from build123d import *

# Parameters (mm, degrees)
SKETCH1_W           = 67
SKETCH1_H           = 30
BOSS_EXTRUDE1_DEPTH = 25
SKETCH2_W           = 57
SKETCH2_H           = 22
CUT_EXTRUDE1_DEPTH  = 17
SKETCH3_R           = 10
SKETCH3_R_2         = 8
SKETCH3_R_3         = 2
CUT_EXTRUDE2_DEPTH  = 8
BOSS_EXTRUDE2_START = -67
SKETCH4_W           = 5
SKETCH4_H           = 15
BOSS_EXTRUDE2_DEPTH = 10
SKETCH4_2_W         = 5
SKETCH4_2_H         = 15
BOSS_EXTRUDE3_DEPTH = 10
SKETCH5_R           = 1.7
CUT_EXTRUDE3_DEPTH  = 10
CUT_EXTRUDE4_DEPTH  = 8
SKETCH8_W           = 67
SKETCH8_H           = 25
BOSS_EXTRUDE4_DEPTH = 50
SKETCH9_W           = 57
SKETCH9_H           = 22
CUT_EXTRUDE6_DEPTH  = 17
SKETCH11_R          = 10
SKETCH11_R_2        = 8
SKETCH11_R_3        = 2
CUT_EXTRUDE7_DEPTH  = 81.039052968
CUT_EXTRUDE8_DEPTH  = 81.039052968
FILLET1_R           = 3


with BuildPart() as part:
    # Sketch1 → Boss-Extrude1 (new body)
    with BuildSketch(Plane(origin=(0, 0, 0), x_dir=(1, 0, 0), z_dir=(0, 1, 0))):
        Rectangle(SKETCH1_W, SKETCH1_H)
    extrude(amount=BOSS_EXTRUDE1_DEPTH)

    # Sketch2 → Cut-Extrude1 (cut)
    with BuildSketch(Plane(origin=(0, 25, 0), x_dir=(1, 0, 0), z_dir=(0, 1, 0))):
        Rectangle(SKETCH2_W, SKETCH2_H)
    extrude(amount=-CUT_EXTRUDE1_DEPTH, mode=Mode.SUBTRACT)

    # Sketch3 → Cut-Extrude2 (cut)
    with BuildSketch(Plane(origin=(0, 8, 0), x_dir=(1, 0, 0), z_dir=(0, 1, 0))):
        with Locations((10, 0)):
            Circle(SKETCH3_R)
        with Locations((-3, 0)):
            Circle(SKETCH3_R_2)
        with Locations(Location((-24.5, 5, 0), (0, 0, 270))):
            Circle(SKETCH3_R_3)
        with Locations(Location((-24.5, -5, 0), (0, 0, 270))):
            Circle(SKETCH3_R_3)
        with Locations(Location((24.5, 5, 0), (0, 0, 270))):
            Circle(SKETCH3_R_3)
        with Locations(Location((24.5, -5, 0), (0, 0, 270))):
            Circle(SKETCH3_R_3)
    extrude(amount=-CUT_EXTRUDE2_DEPTH, mode=Mode.SUBTRACT)

    # Sketch4 → Boss-Extrude2 (add)
    with BuildSketch(Plane(origin=(33.5, 0, 0), x_dir=(0, 0, -1), z_dir=(1, 0, 0)).offset(BOSS_EXTRUDE2_START)):
        with Locations((-12.5, 12.5)):
            Rectangle(SKETCH4_W, SKETCH4_H)
    extrude(amount=-BOSS_EXTRUDE2_DEPTH)

    # Sketch4<2> → Boss-Extrude3 (add)
    with BuildSketch(Plane(origin=(33.5, 0, 0), x_dir=(0, 0, -1), z_dir=(1, 0, 0))):
        with Locations((-12.5, 12.5)):
            Rectangle(SKETCH4_2_W, SKETCH4_2_H)
    extrude(amount=BOSS_EXTRUDE3_DEPTH)

    # Sketch5 → Cut-Extrude3 (cut)
    with BuildSketch(Plane(origin=(0, 0, 10), x_dir=(-1, 0, 0), z_dir=(0, 0, -1))):
        with Locations(Location((38, 12.5, 0), (0, 0, 90))):
            Circle(SKETCH5_R)
        with Locations(Location((-38, 12.5, 0), (0, 0, 90))):
            Circle(SKETCH5_R)
    extrude(amount=-CUT_EXTRUDE3_DEPTH, mode=Mode.SUBTRACT)

    # Sketch6 → Cut-Extrude4 (cut)
    with BuildSketch(Plane(origin=(0, 8, 0), x_dir=(1, 0, 0), z_dir=(0, 1, 0))):
        Polygon((-21, 11.00455557), (-21.003329437, -10.997477388), (10, -11.002168937), (10, 10.997831063), align=None)
    extrude(amount=-CUT_EXTRUDE4_DEPTH, mode=Mode.SUBTRACT)

    # Sketch8 → Boss-Extrude4 (add)
    with BuildSketch(Plane(origin=(0, 0, -15), x_dir=(-1, 0, 0), z_dir=(0, 0, -1))):
        with Locations((0, 12.5)):
            Rectangle(SKETCH8_W, SKETCH8_H)
    extrude(amount=BOSS_EXTRUDE4_DEPTH)

    # Sketch9 → Cut-Extrude6 (cut)
    with BuildSketch(Plane(origin=(0, 25, 0), x_dir=(1, 0, 0), z_dir=(0, 1, 0))):
        with Locations((0, 30)):
            Rectangle(SKETCH9_W, SKETCH9_H)
    extrude(amount=-CUT_EXTRUDE6_DEPTH, mode=Mode.SUBTRACT)

    # Sketch11 → Cut-Extrude7 (cut, through all)
    with BuildSketch(Plane(origin=(0, 8, 0), x_dir=(1, 0, 0), z_dir=(0, 1, 0))):
        with Locations((9.177125898, 30.121191818)):
            Circle(SKETCH11_R)
        with Locations((-3.822874102, 30.121191818)):
            Circle(SKETCH11_R_2)
        with Locations(Location((-25.322874102, 35.121191818, 0), (0, 0, 270))):
            Circle(SKETCH11_R_3)
        with Locations(Location((-25.322874102, 25.121191818, 0), (0, 0, 270))):
            Circle(SKETCH11_R_3)
        with Locations(Location((23.677125898, 35.121191818, 0), (0, 0, 270))):
            Circle(SKETCH11_R_3)
        with Locations(Location((23.677125898, 25.121191818, 0), (0, 0, 270))):
            Circle(SKETCH11_R_3)
    extrude(amount=-CUT_EXTRUDE7_DEPTH, mode=Mode.SUBTRACT)

    # Sketch13 → Cut-Extrude8 (cut, through all)
    with BuildSketch(Plane(origin=(0, 8, 0), x_dir=(1, 0, 0), z_dir=(0, 1, 0))):
        Polygon((-20.928820676, 40.842619331), (-20.932150113, 18.840586374), (10.071179324, 18.835894824), (10.071179324, 40.835894824), align=None)
    extrude(amount=-CUT_EXTRUDE8_DEPTH, mode=Mode.SUBTRACT)

    # Fillet1
    fillet1_edges = [part.edges().sort_by_distance(p)[0] for p in [
        (0, 25, -41),
        (0, 25, -19),
        (0, 25, 11),
        (-43.5, 12.5, 10),
        (-33.5, 20, 12.5),
        (-33.5, 5, 12.5),
        (0, 25, -11),
        (33.5, 20, 12.5),
        (33.5, 5, 12.5),
        (43.5, 12.5, 10),
        (33.5, 12.5, -65),
        (-33.5, 12.5, -65),
    ]]
    fillet(fillet1_edges, radius=FILLET1_R)


solid = part.part
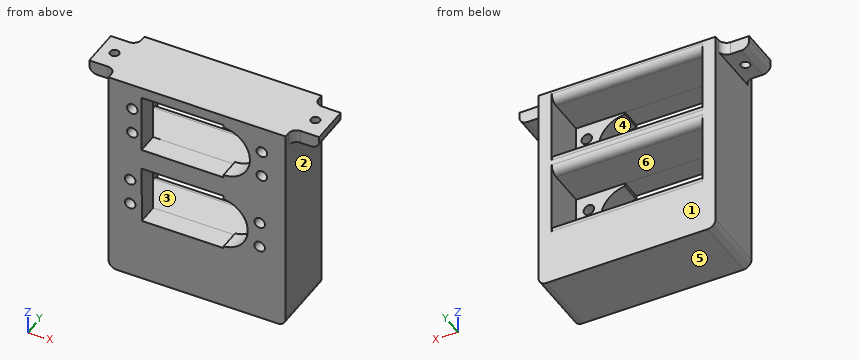
Build history of the part. All positions in model axes, mm. Face numbers are marked on the shaded views. A direction names the side the tool comes from. Round coordinates to 2 decimals unless told otherwise and drop trailing zeros. Loops run counter-clockwise (first coordinate to the right, second up) from the corner with the lowest first, then second, coordinate; pieces in that order, holes last. Notation, with made-up numbers: (50, 36) -> (99, 36) arc R24 cw to (99, 74) -> close; hole circle Ø9 at (-15, 19). An arc over 180 degrees is marked (long way). One line per item, written item: value. Start each with the question number.
Q1. Probe line 1 along Z through (x, y) = (-16, 11.25); line 2 along X through (y, z) = (12.5, 13.55); line 3 along Z through (x, y) = (2.5, 4.5). List the from-to ranges inside material, lowest first.
Q2. Cut at D-D on x = 16.5. List the corners of the cut face in (y, z).
Q3. Cut at B-B on x = -38. List the corners of the cut face in (y, z).
Q4. Cut at C-C on z = -30. List the corners of the cut face in (x, y), plus the area to 3 significant figures.
Q5. Drop flat-ended pins along their axis: pin 1 Ø0.8 at (y, z) = (5, 10.5) entering from -X; pin 2 Ø8.5 at (y, z) = (16.5, -32) entering from +X; pin 3 Ø12 at (y, z) = (3, -55) entering from -X. Give the stop position or say it passes through.
Q6. Cut at A-A on y = 12.5. List the corners of the cut face in (x, z).
Q7. 3-axis set-ups, long thin cutter, end or side, ignore diameter. For the marked faces 4, 5 and 6: which of +Z, -Z, +X, -X, +Y, -Y reach the whole face in a straight line?
Q8. Two-plate mould, pull along X, no slides. Class the marked faces 1, 2 and 3: released by +X, released by -X, zero draft, split by the parting line, or undercut.
Computed:
1. line 1: -65 to -41, -19 to -11, 11 to 15
1. line 2: -43.5 to -39.7, -36.3 to 36.3, 39.7 to 43.5
1. line 3: -65 to -40.84, -18.84 to -11, 11 to 15
2. outline: (0, -65) -> (25, -65) -> (25, -44) arc R3 ccw to (22, -41) -> (8, -41) -> (8, -36.93) -> (0, -36.93) -> close; (0, -23.31) -> (8, -23.31) -> (8, -19) -> (22, -19) arc R3 ccw to (25, -16) -> (25, -14) arc R3 ccw to (22, -11) -> (8, -11) -> (8, -7.6) -> (0, -7.6) -> close; (0, 7.6) -> (8, 7.6) -> (8, 11) -> (22, 11) arc R3 ccw to (25, 14) -> (25, 15) -> (0, 15) -> close
3. outline: (5, 10) -> (10.8, 10) -> (10.8, 15) -> (5, 15) -> close; (14.2, 10) -> (20, 10) -> (20, 15) -> (14.2, 15) -> close
4. outline: (-33.5, 0) -> (-20.93, 0) -> (-20.93, 8) -> (-28.5, 8) -> (-28.5, 25) -> (-33.5, 25) -> close; (19.18, 0) -> (33.5, 0) -> (33.5, 25) -> (28.5, 25) -> (28.5, 8) -> (19.18, 8) -> close
4. area: 385 mm²
5. pin 1: x = -42.64
5. pin 2: x = 33.5
5. pin 3: x = -33.5
6. outline: (-43.5, 13) arc R3 ccw to (-40.5, 10) -> (-39.7, 10) -> (-39.7, 15) -> (-43.5, 15) -> close; (-36.3, 10) -> (-33.5, 10) -> (-33.5, -62) arc R3 ccw to (-30.5, -65) -> (30.5, -65) arc R3 ccw to (33.5, -62) -> (33.5, 10) -> (36.3, 10) -> (36.3, 15) -> (-36.3, 15) -> close; (39.7, 10) -> (40.5, 10) arc R3 ccw to (43.5, 13) -> (43.5, 15) -> (39.7, 15) -> close; hole (-28.5, -41) -> (28.5, -41) -> (28.5, -19) -> (-28.5, -19) -> close; hole (-28.5, -11) -> (28.5, -11) -> (28.5, 11) -> (-28.5, 11) -> close
7. face 4: +Y, -Y
7. face 5: -Z, +X, -X, +Y, -Y
7. face 6: +Y
8. face 1: zero draft
8. face 2: released by +X
8. face 3: undercut
